Geometry check sheet. Reference: the model listing, model coordinates, mm. Face numbers are marked on the shaded views. Give positions to 0.01 mm unless a question says otherwise; leave off trailing zeros. Write each loop counter-clockwise with the first axis right and the second up, starting at its lowest first coordinate (ties: lowest second). Pieces come first, ordered by that corner, then holes. Notation, with made-up numbers: M 83.5,61 L 94.5,61 A17 cw 94.5,75 Z; hole C -11.5,-10.75 d7. An arc over 180 degrees is marked long. Use one line per item in the form item = value. Start each with the question number.
```python
from build123d import *

# Parameters (mm, degrees)
SKETCH1_R                 = 12.5
BOSS_EXTRUDE1_DEPTH       = 119.4
SKETCH4_W                 = 8
SKETCH4_H                 = 8
CUT_EXTRUDE1_DEPTH        = 35.4
SKETCH5_R                 = 15.3
BOSS_EXTRUDE2_DEPTH       = 2
SKETCH10_R                = 12.5
BOSS_EXTRUDE5_DEPTH       = 15
SKETCH14_R                = 12.5
CUT_EXTRUDE3_DEPTH        = 0.53629326
M6X1_0_TAPPED_HOLE2_D     = 5
M6X1_0_TAPPED_HOLE2_DEPTH = 18.497848452
M6X1_0_TAPPED_HOLE2_TIP   = 1.502151548
SKETCH20_R                = 42.5
BOSS_EXTRUDE6_DEPTH       = 5
FILLET3_R                 = 10
M6X1_0_TAPPED_HOLE3_D     = 5
SKETCH23_R                = 20
CUT_EXTRUDE4_DEPTH        = 1.5


with BuildPart() as part:
    # Sketch1 → Boss-Extrude1 (new body)
    with BuildSketch(Plane.XY):
        Circle(SKETCH1_R)
    extrude(amount=BOSS_EXTRUDE1_DEPTH)

    # Sketch4 → Cut-Extrude1 (cut)
    with BuildSketch(Plane(origin=(0, 0, 0), x_dir=(-1, 0, 0), z_dir=(0, 0, -1))):
        with Locations((0, 12.5)):
            Rectangle(SKETCH4_W, SKETCH4_H)
    extrude(amount=-CUT_EXTRUDE1_DEPTH, mode=Mode.SUBTRACT)

    # Sketch5 → Boss-Extrude2 (add)
    with BuildSketch(Plane.XY.offset(119.4)):
        Circle(SKETCH5_R)
    extrude(amount=BOSS_EXTRUDE2_DEPTH)

    # Sketch10 → Boss-Extrude5 (add)
    with BuildSketch(Plane.XY.offset(121.4)):
        with Locations(Location((0, 0, 0), (0, 0, 108.662924885))):
            Circle(SKETCH10_R)
    extrude(amount=BOSS_EXTRUDE5_DEPTH)

    # Sketch14 → Cut-Extrude3 (cut)
    with BuildSketch(Plane(origin=(0, 0, 0), x_dir=(-1, 0, 0), z_dir=(0, 0, -1))):
        with Locations(Location((0, 0, 0), (0, 0, 71.337075115))):
            Circle(SKETCH14_R)
    extrude(amount=-CUT_EXTRUDE3_DEPTH, mode=Mode.SUBTRACT)

    # M6x1.0 Tapped Hole2
    with Locations(Plane(origin=(0, 0, 0.53629326), x_dir=(-1, 0, 0), z_dir=(0, 0, -1))):
        with Locations((0, 0)):
            Hole(M6X1_0_TAPPED_HOLE2_D / 2, depth=M6X1_0_TAPPED_HOLE2_DEPTH)
            with Locations((0, 0, -(M6X1_0_TAPPED_HOLE2_DEPTH + M6X1_0_TAPPED_HOLE2_TIP / 2))):  # 118° drill point
                Cone(0, M6X1_0_TAPPED_HOLE2_D / 2, M6X1_0_TAPPED_HOLE2_TIP, mode=Mode.SUBTRACT)

    # Sketch20 → Boss-Extrude6 (add)
    with BuildSketch(Plane.XY.offset(136.4)):
        Circle(SKETCH20_R)
    extrude(amount=-BOSS_EXTRUDE6_DEPTH)

    # Fillet3
    fillet3_edges = [part.edges().sort_by_distance(p)[0] for p in [
        (4, -11.842719282, 131.4),
    ]]
    fillet(fillet3_edges, radius=FILLET3_R - 0.0001)  # a hair under: the kernel refuses the full size

    # M6x1.0 Tapped Hole3 (through all)
    with Locations(Plane.XY.offset(136.4)):
        with Locations((0, 36), (36, 0), (0, -36), (-36, 0)):
            Hole(M6X1_0_TAPPED_HOLE3_D / 2)

    # Sketch23 → Cut-Extrude4 (cut)
    with BuildSketch(Plane.XY.offset(136.4)):
        Circle(SKETCH23_R)
    extrude(amount=-CUT_EXTRUDE4_DEPTH, mode=Mode.SUBTRACT)


solid = part.part
```
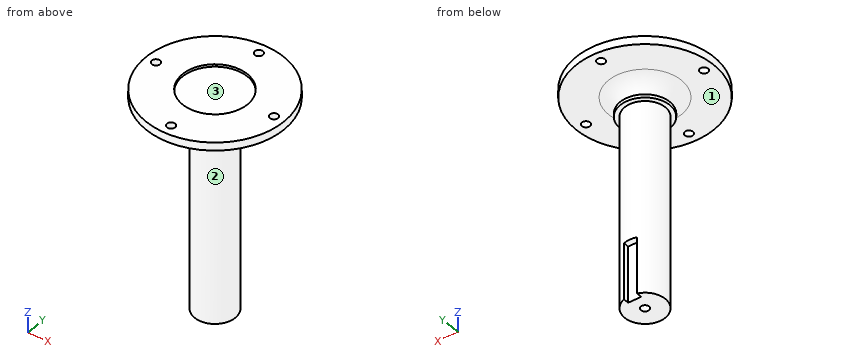
(1) Thickness scan on probe 1 along Y at (x, z) = (0, 135); probe 2 along Y at (x, z) = (0, 132.75); probe 3 along X at (y, z) = (0, 13.25). Record the ranges inside material, lowest first. Write a range as [from, to].
(2) Depth check by flat-ended pin: pin 1 (12 mm diameter, centred on x = 1.5, z = 50, fed in from +Y); pin 2 (24 mm diameter, centred on x = 0, y = 0, fed in from +Z); pin 3 (9 mm diameter, centred on x = 1.5, z = 26.5, fed in from +Y); pin 4 (4 mm diameter, centred on x = 36, y = 0, fed in from -Z). Enter the tip coordinate at first touch or a pass-through.
(3) Sectioned sample at B-B, the plane y = -36. Record the boundary of the cut face in (x, z).
(4) Sectioned sample at D-D, the plane z = 30. Record the boundary of the cut face in (x, y), plus the area to 3 significant figures.
(5) Sectioned sample at C-C, the plane z = 98. Record the boundary of the cut face in (x, y), plus the area to 3 significant figures.
(6) Draft check along X on the marked faces 1, 2 and 3. Enter one of: released by +X, released by -X, zero draft, split by the parting line, or undercut.
(7) Sectioned sample at A-A, the plane x = -36.5. Record the boundary of the cut face in (y, z), plus the area to 3 significant figures.
Numbers:
q1.probe_1 = [-42.5, -38.5], [-33.5, -20], [20, 33.5], [38.5, 42.5]
q1.probe_2 = [-42.5, -38.5], [-33.5, 33.5], [38.5, 42.5]
q1.probe_3 = [-12.5, -2.5], [2.5, 12.5]
q2.pin_1 = 12.5
q2.pin_2 = 134.9
q2.pin_3 = 11.84
q2.pin_4 = through
q3.outline = M -22.59,131.4 L -2.5,131.4 L -2.5,136.4 L -22.59,136.4 Z; M 2.5,131.4 L 22.59,131.4 L 22.59,136.4 L 2.5,136.4 Z
q4.outline = M -4,8.5 L -4,11.84 A12.5 ccw long 4,11.84 L 4,8.5 Z
q4.area = 461 mm2
q5.outline = C 0,0 d25
q5.area = 491 mm2
q6.face_1 = zero draft
q6.face_2 = split by the parting line
q6.face_3 = undercut
q7.outline = M -21.77,131.4 L -2.45,131.4 L -2.45,136.4 L -21.77,136.4 Z; M 2.45,131.4 L 21.77,131.4 L 21.77,136.4 L 2.45,136.4 Z
q7.area = 193 mm2
